Source: three-view drawing plus pictorial views. Frame: mm from the lowest corner of the part. Coordinates: 2 decimals unless noted, no trailing zeros. Loops run counter-clockwise (first coordinate to the right, second up) from the corner with the lowest first, then second, coordinate; pieces in that order, holes last.
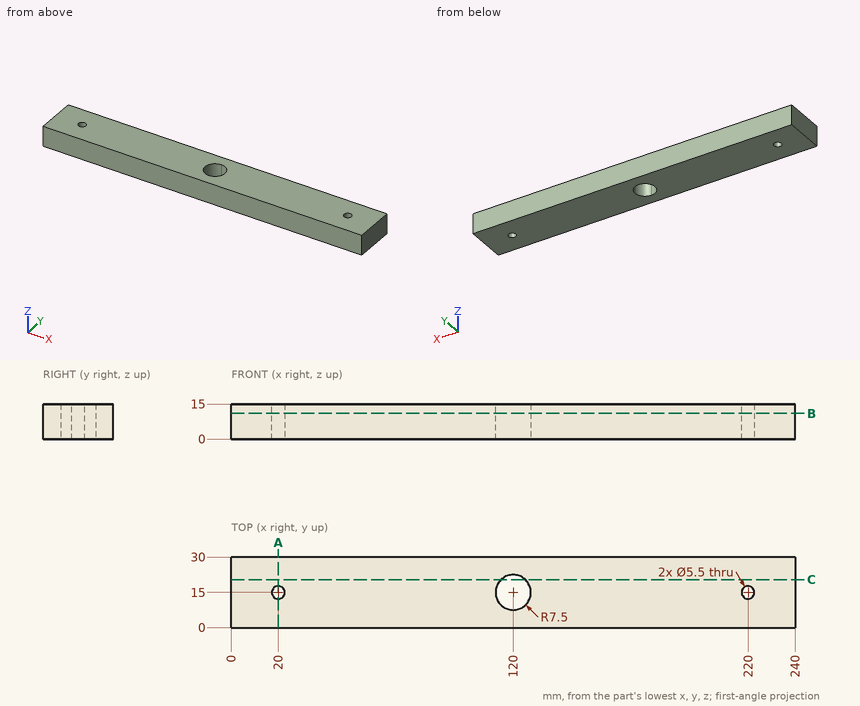
Q1. Section B-B, the plane z = 11. Return the cut outline in (x, y), plus the area to 3 significant figures.
Q2. Section C-C, the plane y = 20.5. Return the cut outline in (x, z), plus the area to 3 significant figures.
Q3. Section A-A, the plane x = 20. Return the cut outline in (y, z).
Q4. Line query: line 1 along X through (y, z) = (14.75, 7); line 2 along Y through (x, z) = (20, 5.25); line 3 along X through (y, z) = (12.5, 9.5). Output: solid intervals per line, ascending.
Derived:
1. outline: (0, 0) - (240, 0) - (240, 30) - (0, 30) - close; hole circle Ø5.5 at (20, 15); hole circle Ø15 at (120, 15); hole circle Ø5.5 at (220, 15)
1. area: 6,980 mm2
2. outline: (0, 0) - (114.9, 0) - (114.9, 15) - (0, 15) - close; (125.1, 0) - (240, 0) - (240, 15) - (125.1, 15) - close
2. area: 3,450 mm2
3. outline: (0, 0) - (12.25, 0) - (12.25, 15) - (0, 15) - close; (17.75, 0) - (30, 0) - (30, 15) - (17.75, 15) - close
4. line 1: x = 0 to 17.26, 22.74 to 112.5, 127.5 to 217.26, 222.74 to 240
4. line 2: y = 0 to 12.25, 17.75 to 30
4. line 3: x = 0 to 18.85, 21.15 to 112.93, 127.07 to 218.85, 221.15 to 240
